Geometry check sheet. Reference: the model listing, model coordinates, mm. A direction names the side the tool comes from. Round coordinates to 2 decimals unless told otherwise and drop trailing zeros. Write each loop counter-clockwise with the first axis right and the second up, starting at its lowest first coordinate (ties: lowest second). Pieces come first, ordered by that corner, then holes.
from build123d import *

# Parameters (mm, degrees)
F1_START = 70
F0_R     = 27.5
F0_R_2   = 21.5
F0_R_3   = 1.5
F1_DEPTH = 200
F2_START = 40
F2_DEPTH = 30
F3_DEPTH = 40
F3_TAPER = -15
F4_R     = 11.3468037432


with BuildPart() as f1:
    # F0 (on Top) → F1 (new body)
    with BuildSketch(Plane.XY.offset(F1_START)):
        with Locations((22.4150829017, 24.535804987)):
            Circle(F0_R)
        with Locations((22.4150829017, 24.535804987)):
            Circle(F0_R_2, mode=Mode.SUBTRACT)
        with Locations((22.4150829017, 24.535804987)):
            Circle(F0_R_2)
        with Locations((22.4150829017, 24.535804987)):
            Circle(F0_R_3, mode=Mode.SUBTRACT)
        with Locations((22.4150829017, 24.535804987)):
            Circle(F0_R_3)
    extrude(amount=F1_DEPTH)

    # F0 (on Top) → F2 (join)
    with BuildSketch(Plane.XY.offset(F2_START)):
        with Locations((22.4150829017, 24.535804987)):
            Circle(F0_R_2)
        with Locations((22.4150829017, 24.535804987)):
            Circle(F0_R_3, mode=Mode.SUBTRACT)
        with Locations((22.4150829017, 24.535804987)):
            Circle(F0_R_3)
    extrude(amount=F2_DEPTH)

    # F0 (on Top) → F3 (join)
    with BuildSketch(Plane.XY):
        with Locations((22.4150829017, 24.535804987)):
            Circle(F0_R_3)
    extrude(amount=F3_DEPTH, taper=F3_TAPER)

    # F4
    f4_edges = [f1.edges().sort_by_distance(p)[0] for p in [
        (-5.084917, 24.535805, 270),
    ]]
    fillet(f4_edges, radius=F4_R)


solid = f1.part
1. Depth check by flat-ended pin: pin 1 Ø3 at (x, z) = (4, 126.5) entering from +Y; pin 2 Ø1 at (y, z) = (23, 145) entering from +X; pin 3 Ø6 at (x, y) = (2.5, 22) entering from -Z. Enter the tip coordinate at first touch or a pass-through.
2. Section check B-B (z = 66.5). Record the cut outline in (x, y).
3. Section check A-A (z = 188). Record the cut outline in (x, y), plus the area to 3 significant figures.
4. Access from +Z, -Z, +X, -X, +Y, -Y to the whole of each face (thin tool, end or side, straight path). Record for faces 1 (the face through (22, 25, 270)), 2 (the face through (6, 10, 70)).
5. Scan lines: line 1 along X through (y, z) = (23.5, 193); line 2 along Z through (x, y) = (36.5, 37.5); line 3 along X through (y, z) = (26.5, 189). Record each from-to range of solid material in increasing order.
Results below:
1. pin 1: stops at y = 46.22
1. pin 2: stops at x = 49.9
1. pin 3: stops at z = 40
2. outline: circle Ø43 at (22.42, 24.54)
3. outline: circle Ø55 at (22.42, 24.54)
3. area: 2,380 mm2
4. face 1: +Z, +X, -X, +Y, -Y
4. face 2: -Z
5. line 1: x = -5.07 to 49.9
5. line 2: z = 40 to 269.6
5. line 3: x = -5.01 to 49.84
